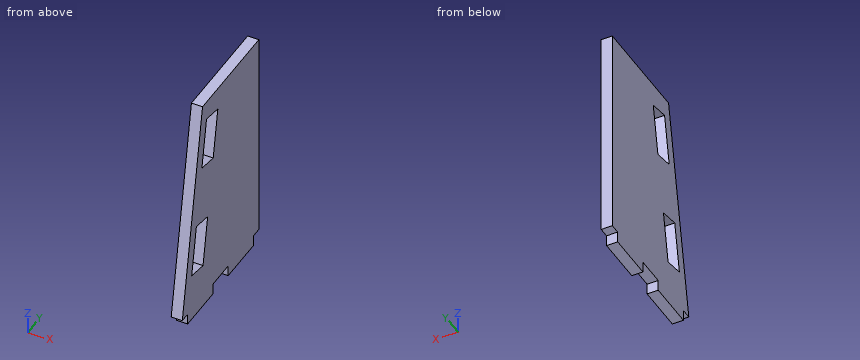
```python
from build123d import *

# Parameters (mm, degrees)
F0_W     = 83.82
F0_H     = 19.558
F1_DEPTH = 19.558


with BuildPart() as f1:
    # F0 (on Right) → F1 (new body)
    with BuildSketch(Plane.YZ):
        Polygon((-17.953301, 168.605641), (-85.133881, -212.394359), (-67.353881, -212.394359), (-17.953301, -212.394359), (16.466119, -212.394359), (67.266119, -212.394359), (151.086119, -212.394359), (168.866119, -212.394359), (168.866119, 168.605641), align=None)
        Polygon((-0.928284, -63.954421), (-16.365607, -151.50383), (-53.886782, -144.887834), (-38.449459, -57.338425), align=None, mode=Mode.SUBTRACT)
        Polygon((32.874382, 127.750025), (17.437059, 40.200616), (-20.084116, 46.816611), (-4.646793, 134.366021), align=None, mode=Mode.SUBTRACT)
        Polygon((-17.953301, -212.394359), (-67.353881, -212.394359), (-67.353881, -231.952359), (16.466119, -231.952359), (16.466119, -212.394359), align=None)
        with Locations((109.176119, -222.173359)):
            Rectangle(F0_W, F0_H)
    extrude(amount=F1_DEPTH)


solid = f1.part
```
Geometry: final body of the model. Coordinates: model frame, mm. Coordinates: 2 decimals unless noted, no trailing zeros. Loops run counter-clockwise (first coordinate to the right, second up) from the corner with the lowest first, then second, coordinate; pieces in that order, holes last. Notation, with made-up numbers: M 84.25,-33 L 91.25,-33 A13 ccw 91.25,-11 Z; hole C 14.25,-23 d10. An arc over 180 degrees is marked long. Put each result on its own line as item: value.
(1) First-contact query: pin 1 (9 mm diameter, centred on x = 13, y = -73, fed in from -Z); pin 2 (1.5 mm diameter, centred on x = 9, z = 97.5, fed in from -Y); pin 3 (6 mm diameter, centred on x = 9, z = -222, fed in from -Y); pin 4 (1 mm diameter, centred on y = -17.5, z = 67, fed in from -X). Flat tips, straight axial feed; report the tip coordinate or a pass-through.
Answer sheet:
pin 1: stops at z = -212.39
pin 2: stops at y = -30.62
pin 3: stops at y = -67.35
pin 4: stops at x = 0
(2) Cut plane B-B on z = 110. Return the cut outline in (x, y).
Answer sheet:
outline: M 0,-28.29 L 19.56,-28.29 L 19.56,-8.94 L 0,-8.94 Z; M 0,29.74 L 19.56,29.74 L 19.56,168.87 L 0,168.87 Z
(3) Material intervals for probe 1 along Y at (x, z) = (18.75, 96); probe 2 along Y at (x, z) = (12.75, 47); probe 3 along Y at (x, z) = (7.5, 32), sorted ascending.
Answer sheet:
probe 1: y = -30.76 to -11.41, 27.28 to 168.87
probe 2: y = -39.4 to -20.05, 18.64 to 168.87
probe 3: y = -42.04 to 168.87
(4) Cut plane A-A on x = 5.5. Return the cut outline in (y, z).
Answer sheet:
outline: M -85.13,-212.39 L -67.35,-212.39 L -67.35,-231.95 L 16.47,-231.95 L 16.47,-212.39 L 67.27,-212.39 L 67.27,-231.95 L 151.09,-231.95 L 151.09,-212.39 L 168.87,-212.39 L 168.87,168.61 L -17.95,168.61 Z; hole M -53.89,-144.89 L -16.37,-151.5 L -0.93,-63.95 L -38.45,-57.34 Z; hole M -20.08,46.82 L 17.44,40.2 L 32.87,127.75 L -4.65,134.37 Z
(5) Cut plane C-C on z = 67. Return the cut outline in (x, y).
Answer sheet:
outline: M 0,-35.87 L 19.56,-35.87 L 19.56,-16.53 L 0,-16.53 Z; M 0,22.16 L 19.56,22.16 L 19.56,168.87 L 0,168.87 Z
(6) Cut plane D-D on z = -50.5. Return the cut outline in (x, y), then the cut area to 3 significant figures.
Answer sheet:
outline: M 0,-56.59 L 19.56,-56.59 L 19.56,168.87 L 0,168.87 Z
area: 4,410 mm^2
